Geometry check sheet. Reference: the model listing, model coordinates, mm. Round coordinates to 2 decimals unless told otherwise and drop trailing zeros. Write each loop counter-clockwise with the first axis right and the second up, starting at its lowest first coordinate (ties: lowest second). Pieces come first, ordered by that corner, then holes. Notation, with made-up numbers: (69, 35.5) -> (100, 35.5) arc R35 ccw to (100, 67.5) -> close; hole circle Ø9 at (65.25, -36). An arc over 180 degrees is marked (long way). Return JSON: item names as keys, results as strings. Group by question number.
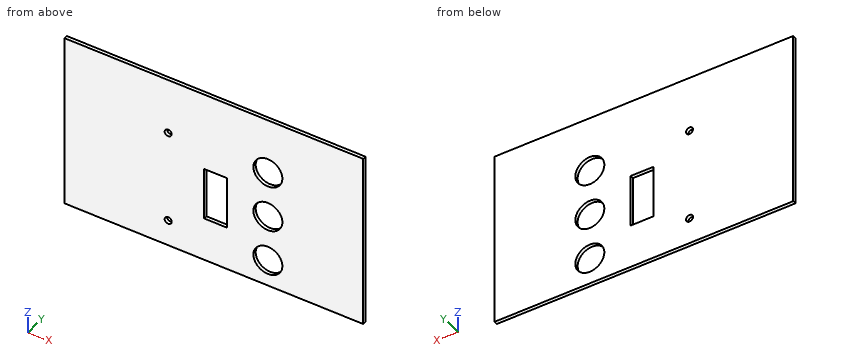
from build123d import *

# Parameters (mm, degrees)
F0_W     = 170
F0_H     = 100
F1_DEPTH = 2
F2_R     = 8.25
F2_W     = 13
F2_H     = 30
F2_R_2   = 2
F3_DEPTH = 25


with BuildPart() as f1:
    # F0 (on Front) → F1 (new body)
    with BuildSketch(Plane.XZ):
        Rectangle(F0_W, F0_H)
    extrude(amount=F1_DEPTH)

    # F2 (on face) → F3 (cut)
    with BuildSketch(Plane.XZ.offset(2)):
        with Locations((30.75, -34.75)):
            Circle(F2_R)
        with Locations((30.75, -8.25)):
            Circle(F2_R)
        with Locations((30.75, 18.25)):
            Circle(F2_R)
        with Locations((1, -10)):
            Rectangle(F2_W, F2_H)
        with Locations((-26, -35)):
            Circle(F2_R_2)
        with Locations((-26, 18)):
            Circle(F2_R_2)
    extrude(amount=-F3_DEPTH, mode=Mode.SUBTRACT)


solid = f1.part
1) Sectioned sample at C-C on x = -26. Enter the section's corners in (y, z), and give its area (3 significant figures).
2) Sectioned sample at A-A on y = -0.6. Enter the section's corners in (x, z).
3) Go/stop test with a flat-tipped pin: P1, Ø3, axis at x = -26, z = -35, coming from the +Y side. Record where the tip stops, or that it passes through.
4) Material ranges on probe 1 along Z at (x, y) = (-26, -1.65); probe 2 along Z at (x, y) = (3, -1.2); probe 3 along X at (y, z) = (-1.4, -2.5), recorded low to high. Write a range as [from, to].
5) Sectioned sample at B-B on x = 30.75. Enter the section's corners in (y, z).
Evaluation:
{
 "1": {"outline": "(-2, -50) -> (0, -50) -> (0, -37) -> (-2, -37) -> close; (-2, -33) -> (0, -33) -> (0, 16) -> (-2, 16) -> close; (-2, 20) -> (0, 20) -> (0, 50) -> (-2, 50) -> close", "area": "184 mm2"},
 "2": {"outline": "(-85, -50) -> (85, -50) -> (85, 50) -> (-85, 50) -> close; hole circle Ø4 at (-26, -35); hole circle Ø4 at (-26, 18); hole (-5.5, -25) -> (7.5, -25) -> (7.5, 5) -> (-5.5, 5) -> close; hole circle Ø16.5 at (30.75, -34.75); hole circle Ø16.5 at (30.75, -8.25); hole circle Ø16.5 at (30.75, 18.25)"},
 "3": {"P1": "passes through"},
 "4": {"probe 1": "z = [-50, -37], [-33, 16], [20, 50]", "probe 2": "z = [-50, -25], [5, 50]", "probe 3": "x = [-85, -5.5], [7.5, 24.83], [36.67, 85]"},
 "5": {"outline": "(-2, -50) -> (0, -50) -> (0, -43) -> (-2, -43) -> close; (-2, -26.5) -> (0, -26.5) -> (0, -16.5) -> (-2, -16.5) -> close; (-2, 0) -> (0, 0) -> (0, 10) -> (-2, 10) -> close; (-2, 26.5) -> (0, 26.5) -> (0, 50) -> (-2, 50) -> close"}
}
